Check sheet for the modelled part. Datum: model origin and axes. Units: mm. Face numbers are marked on the shaded views. A direction names the side the tool comes from. Give positions to 0.01 mm unless a question says otherwise; leave off trailing zeros. Order: outer loops, then holes, each group sorted by start corner. A loop starts at its lowest first (then second) coordinate and runs counter-clockwise, first axis right, second up.
from build123d import *

# Parameters (mm, degrees)
F0_W        = 14.5
F0_H        = 21
F1_DEPTH    = 3
F2_R        = 1.5
F3_DEPTH    = 25
F4_R        = 2.5
F5_W        = 3.125
F5_H        = 5
F6_DEPTH    = 12.5
F7_W        = 14.5
F7_H        = 12
F8_DEPTH    = 3.5
F9_T1_DEPTH = 19.6433659759
F9_T3_DEPTH = 23.5630770458
F10_SIZE    = 0.5


# Not quite as in the source:
# - a fillet or chamfer that OpenCascade refuses, or shapes differently, is made with other operations: its cross-section is extruded or revolved along the edge and cut away or added


with BuildPart() as f1:
    # F0 (on Top) → F1 (new body, symmetric)
    with BuildSketch(Plane.XY):
        Rectangle(F0_W, F0_H)
    extrude(amount=F1_DEPTH, both=True)

    # F2 (on Right) → F3 (cut, symmetric)
    with BuildSketch(Plane.YZ):
        with Locations((-8, 0)):
            Circle(F2_R)
    extrude(amount=F3_DEPTH, both=True, mode=Mode.SUBTRACT)

    # F4
    f4_edges = [f1.edges().sort_by_distance(p)[0] for p in [
        (0, -10.5, 3),
        (0, -10.5, -3),
        (0, 10.5, 3),
        (0, 10.5, -3),
    ]]
    fillet(f4_edges, radius=F4_R)

    # F5 (on Top) → F6 (cut, symmetric)
    with BuildSketch(Plane.XY):
        with Locations((-2.9375, -8)):
            Rectangle(F5_W, F5_H)
        with Locations((2.9375, -8)):
            Rectangle(F5_W, F5_H)
    extrude(amount=F6_DEPTH, both=True, mode=Mode.SUBTRACT)

    # F7 (on face) → F8 (cut)
    with BuildSketch(Plane(origin=(0, 0, -3), x_dir=(1, 0, 0), z_dir=(0, 0, -1))):
        with Locations((0, -2)):
            Rectangle(F7_W, F7_H)
    extrude(amount=-F8_DEPTH, mode=Mode.SUBTRACT)

    # F9: chamfer of 1 on 2 edges, made by hand

    # F9_s2 → F9_t1 (cut)
    with BuildSketch(Plane.YZ.offset(-9.821682988)):
        Polygon((-5, -3), (-4, -2), (-4, -3), align=None)
    extrude(amount=F9_T1_DEPTH, mode=Mode.SUBTRACT)

    # F9_s4 → F9_t3 (cut)
    with BuildSketch(Plane.YZ.offset(-11.7815385229)):
        with BuildLine():
            Line((9.6666666667, -2.3633899812), (8, -1.6180339887))
            Line((8, -1.6180339887), (8, -3))
            ThreePointArc((8, -3), (8.906095825, -2.8300193896), (9.6666666667, -2.3633899812))
        make_face()
    extrude(amount=F9_T3_DEPTH, mode=Mode.SUBTRACT)

    # F10
    f10_edges = [f1.edges().sort_by_distance(p)[0] for p in [
        (-7.25, 0, 3),
        (-4.5, -6.75, 3),
        (-1.375, -6.75, 3),
        (1.375, -6.75, 3),
        (4.5, -6.75, 3),
        (7.25, 0, 3),
        (2.9375, -5.5, 3),
        (-2.9375, -5.5, 3),
        (-7.25, 10.5, 0),
        (7.25, 10.5, 0),
        (-7.25, 9.767767, 2.267767),
        (-7.25, -9.767767, 2.267767),
        (-7.25, -10.5, 0),
        (-7.25, -9.767767, -2.267767),
        (-7.25, -6.5, -3),
        (-7.25, 10.282177, -1.520621),
        (7.25, 10.282177, -1.520621),
        (7.25, 9.767767, 2.267767),
        (7.25, -9.767767, -2.267767),
        (7.25, -10.5, 0),
        (7.25, -9.767767, 2.267767),
        (7.25, -6.5, -3),
        (-4.5, -9.767767, 2.267767),
        (-4.5, -10.5, 0),
        (-4.5, -9.767767, -2.267767),
        (4.5, -6.75, -3),
        (1.375, -6.75, -3),
        (-1.375, -6.75, -3),
        (-4.5, -6.75, -3),
        (4.5, -9.767767, -2.267767),
        (4.5, -10.5, 0),
        (4.5, -9.767767, 2.267767),
        (1.375, -9.767767, 2.267767),
        (1.375, -10.5, 0),
        (1.375, -9.767767, -2.267767),
        (-1.375, -9.767767, 2.267767),
        (-1.375, -10.5, 0),
        (-1.375, -9.767767, -2.267767),
    ]]
    chamfer(f10_edges, length=F10_SIZE)


solid = f1.part
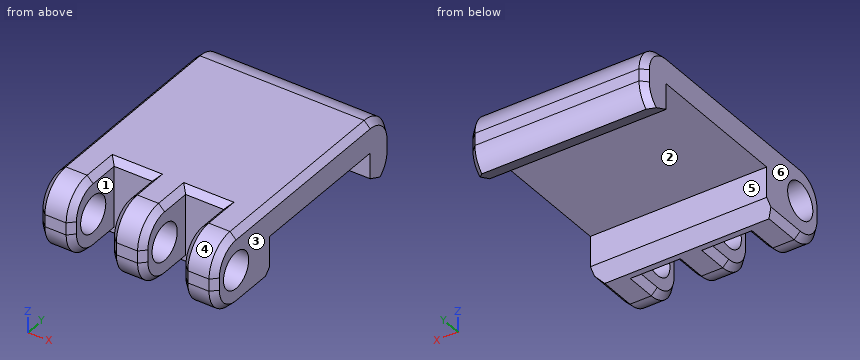
1) Material ranges on L1, parallel to X at y = -7.5, z = -1.5 (3 decimals); L2, parallel to Z at x = 6, y = -8; L3, parallel to Y at x = 5.5, z = -0.75, recorded low to high.
Recorded:
L1: x = -7.25 to -4.5, -1.375 to 1.375, 4.5 to 7.25
L2: z = -3 to -1.5, 1.5 to 3
L3: y = -10.49 to -9.3, -6.7 to -4, 8 to 10.49
2) Draft check along Y on the marked faces 4, 5 and 6. Enter one of: +Y half, -Y half, draft (parallel to the pull), parting line (faces both ways), or undercut.
Recorded:
face 4: -Y half
face 5: undercut
face 6: draft
3) Section check A-A, the plane x = 0.5. Record the cut outline in (y, z).
Recorded:
outline: (-10.5, -0.5) arc R2.5 ccw to (-8, -3) - (-5, -3) - (-4, -2) - (-4, 0.5) - (8, 0.5) - (8, -1.62) - (9.67, -2.36) arc R2.5 ccw to (10.5, -0.5) - (10.5, 0.5) arc R2.5 ccw to (8, 3) - (-8, 3) arc R2.5 ccw to (-10.5, 0.5) - close; hole circle Ø3 at (-8, 0)
4) Section check D-D, the plane y = -5.25. Record the cut outline in (x, z) (3 decimals), then the cut area to 3 significant figures.
Recorded:
outline: (-7.25, -2.5) - (-6.75, -3) - (6.75, -3) - (7.25, -2.5) - (7.25, 2.5) - (6.75, 3) - (5, 3) - (4.75, 2.75) - (1.125, 2.75) - (0.875, 3) - (-0.875, 3) - (-1.125, 2.75) - (-4.75, 2.75) - (-5, 3) - (-6.75, 3) - (-7.25, 2.5) - close
area: 84.6 mm2
5) Section check B-B, the plane z = 0. State how many separate pieces and enclosed holes the cut face has, then the cut area to 3 significant figures.
Recorded:
separate pieces: 5
enclosed holes: 0
area: 73.5 mm2
6) Depth check by flat-ended pin: pin 1 Ø3.5 at (x, z) = (-3.5, -0.5) entering from -Y; pin 2 Ø3 at (x, z) = (3.5, 1.5) entering from -Y. Enter the tip coordinate at first touch or a pass-through.
Recorded:
pin 1: stops at y = -10.5
pin 2: stops at y = -10.37
7) Set-up check for the marked faces 1, 2 and 3: record each of +Z, -Z, +X, -X, +Y, -Y from which the full face is reachable in a straight line by a thin tool's end or side.
Recorded:
face 1: +Z, -Z, -Y
face 2: -Z, +X, -X
face 3: +Z, -Z, +X, +Y, -Y
8) Section check C-C, the plane x = -2.25. Record the cut outline in (y, z), then the cut area to 3 significant figures.
Recorded:
outline: (-5.5, -3) - (-5, -3) - (-4, -2) - (-4, 0.5) - (8, 0.5) - (8, -1.62) - (9.67, -2.36) arc R2.5 ccw to (10.5, -0.5) - (10.5, 0.5) arc R2.5 ccw to (8, 3) - (-5, 3) - (-5.5, 2.5) - close
area: 49.3 mm2
